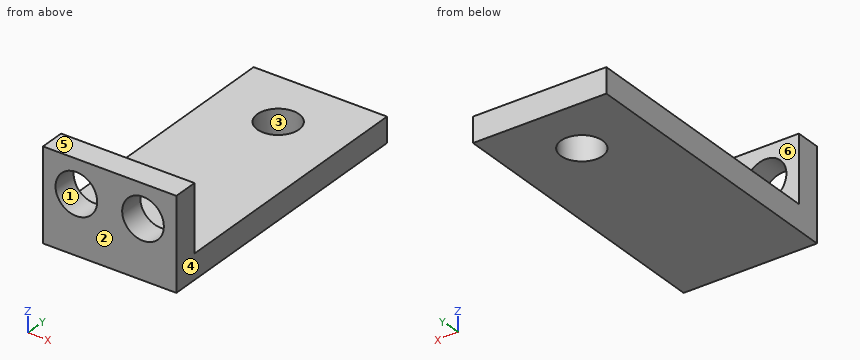
from build123d import *

# Parameters (mm, degrees)
SKETCH1_W           = 16
SKETCH1_H           = 3
BOSS_EXTRUDE1_DEPTH = 35
SKETCH1_3_W         = 16
SKETCH1_3_H         = 11
SKETCH1_3_R         = 2.5
BOSS_EXTRUDE2_DEPTH = 3
SKETCH2_R           = 2.5
CUT_EXTRUDE1_DEPTH  = 8


with BuildPart() as part:
    # Sketch1 → Boss-Extrude1 (new body)
    with BuildSketch(Plane(origin=(0, 0, 0), x_dir=(1, 0, 0), z_dir=(0, 1, 0))):
        with Locations((0, 4)):
            Rectangle(SKETCH1_W, SKETCH1_H)
    extrude(amount=BOSS_EXTRUDE1_DEPTH)

    # Sketch1_3 → Boss-Extrude2 (add)
    with BuildSketch(Plane(origin=(0, 0, 0), x_dir=(1, 0, 0), z_dir=(0, 1, 0))):
        Rectangle(SKETCH1_3_W, SKETCH1_3_H)
        with Locations((4, -1.5)):
            Circle(SKETCH1_3_R, mode=Mode.SUBTRACT)
        with Locations((-4, -1.5)):
            Circle(SKETCH1_3_R, mode=Mode.SUBTRACT)
    extrude(amount=BOSS_EXTRUDE2_DEPTH)

    # Sketch2 → Cut-Extrude1 (cut)
    with BuildSketch(Plane.XY.offset(-2.5)):
        with Locations((0, 28)):
            Circle(SKETCH2_R)
    extrude(amount=-CUT_EXTRUDE1_DEPTH, mode=Mode.SUBTRACT)


solid = part.part
The listing builds one solid part. Answer for the finished solid, in the listing's coordinates (mm). Face numbers are marked on the shaded views. A direction names the side the tool comes from. Round coordinates to 2 decimals unless told otherwise and drop trailing zeros. Write each loop counter-clockwise with the first axis right and the second up, starting at its lowest first coordinate (ties: lowest second). Pieces come first, ordered by that corner, then holes. Notation, with made-up numbers: M 26.25,20 L 71.25,20 A34 ccw 71.25,51 Z; hole C 55,-22.5 d7. An arc over 180 degrees is marked long. Write each question's results on one line, items separated by ' | '. Start each with the question number.
Item 1: Find section D-D on z = -4.5. Write down the section's boundary in (x, y).
Item 2: Given pin 1 Ø8 at (x, y) = (2, 14) entering from +Z; pin 2 Ø6.5 at (x, z) = (-4, 1.5) entering from -Y; pin 3 Ø4 at (x, z) = (4, 1.5) entering from -Y, each flat-ended and moving along its own axis, determine where each tip first touches the part or whether it passes through.
Item 3: Straight lines are drawn through the part: probe 1 along X at (y, z) = (1.2, 1.5); probe 2 along X at (y, z) = (26, -5); probe 3 along Y at (x, z) = (0, -3.75). For each, find the intervals that lie inside material, in ascending order.
Item 4: The mould has two halves that part along X. Classify the marked faces 1, 2, 3 and 4: +X half, -X half, draft (parallel to the pull), parting line (faces both ways), or undercut.
Item 5: Find section A-A on z = 1.5. Write down the section's boundary in (x, y).
Item 6: Find section B-B on x = -5.5. Write down the section's boundary in (y, z).
Item 7: Find section C-C on y = 28. Write down the section's boundary in (x, z), and give its area (3 significant figures).
Item 8: Which of the six approach directions +Z, -Z, +X, -X, +Y, -Y give full straight-line access (tool end or side, diameter ignored) to the marked faces 5 and 6?
Answer block:
1) outline: M -8,0 L 8,0 L 8,35 L -8,35 Z; hole C 0,28 d5
2) pin 1: stops at z = -2.5 | pin 2: stops at y = 0 | pin 3: passes through
3) probe 1: x = -8 to -6.5, -1.5 to 1.5, 6.5 to 8 | probe 2: x = -8 to -1.5, 1.5 to 8 | probe 3: y = 0 to 25.5, 30.5 to 35
4) face 1: undercut | face 2: draft | face 3: undercut | face 4: +X half
5) outline: M -8,0 L -6.5,0 L -6.5,3 L -8,3 Z; M -1.5,0 L 1.5,0 L 1.5,3 L -1.5,3 Z; M 6.5,0 L 8,0 L 8,3 L 6.5,3 Z
6) outline: M 0,-5.5 L 35,-5.5 L 35,-2.5 L 3,-2.5 L 3,-0.5 L 0,-0.5 Z; M 0,3.5 L 3,3.5 L 3,5.5 L 0,5.5 Z
7) outline: M -8,-5.5 L -2.5,-5.5 L -2.5,-2.5 L -8,-2.5 Z; M 2.5,-5.5 L 8,-5.5 L 8,-2.5 L 2.5,-2.5 Z | area: 33.0 mm²
8) face 5: +Z, +X, -X, +Y, -Y | face 6: +Z, +X, -X, +Y
